Check sheet for the drawn part. Datum: minimum x, y, z corner. Units: mm. Coordinates: 2 decimals unless noted, no trailing zeros. Write each loop counter-clockwise with the first axis right and the second up, starting at its lowest first coordinate (ties: lowest second). Pieces come first, ordered by that corner, then holes. Notation, with made-up numbers: M 40.5,76.5 L 53.5,76.5 A19 cw 53.5,83.5 Z; hole C 12.5,33.25 d1. An arc over 180 degrees is marked long. Answer as a JSON object with one key per item and string values. Group by question number.
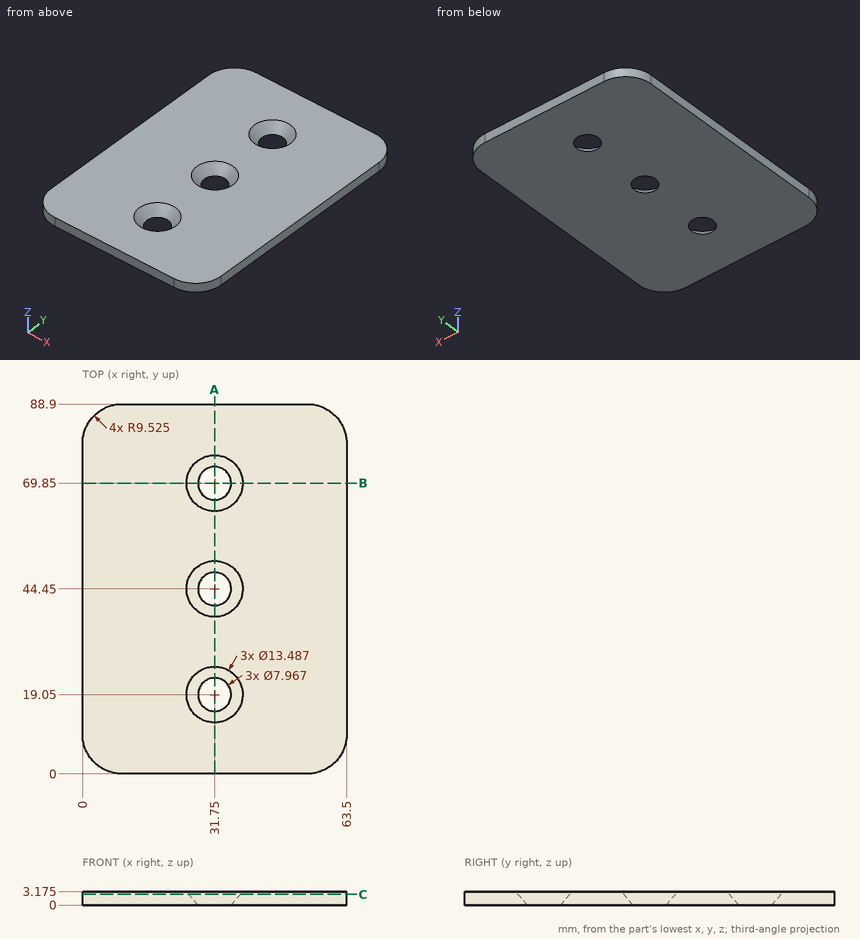
1) Section check C-C (z = 2.55). State how many separate pieces and enclosed holes the cut face has, then the cut area to 4 significant figures.
2) Material ranges on probe 1 along Y at (x, z) = (29, 2.55) (1 decimal); probe 2 along X at (y, z) = (40, 1.1) (1 decimal); probe 3 along X at (y, z) = (74, 2.2), recorded low to high. Write a range as [from, to].
3) Section check A-A (x = 31.75). Record the cut outline in (y, z) (1 decimal), then the cut area to 3 significant figures.
4) Section check B-B (y = 69.85). Record the cut outline in (x, z) (1 decimal).
5) Go/stop test with a flat-tipped pin: pin 1 Ø2 at (x, y) = (26.5, 19) entering from +Z. Record where the tip stops, or that it passes through.
Entries:
{
 "1": {"separate pieces": "1", "enclosed holes": "3", "area": "5,205 mm^2"},
 "2": {"probe 1": "[0, 13.5], [24.6, 38.9], [50, 64.3], [75.4, 88.9]", "probe 2": "[0, 29.6], [33.9, 63.5]", "probe 3": "[0, 27.56], [35.94, 63.5]"},
 "3": {"outline": "M 0,0 L 15.1,0 L 12.3,3.2 L 0,3.2 Z; M 23,0 L 40.5,0 L 37.7,3.2 L 25.8,3.2 Z; M 48.4,0 L 65.9,0 L 63.1,3.2 L 51.2,3.2 Z; M 73.8,0 L 88.9,0 L 88.9,3.2 L 76.6,3.2 Z", "area": "180 mm^2"},
 "4": {"outline": "M 0,0 L 27.8,0 L 25,3.2 L 0,3.2 Z; M 35.7,0 L 63.5,0 L 63.5,3.2 L 38.5,3.2 Z"},
 "5": {"pin 1": "z = 2.61"}
}
